```python
from build123d import *

# Parameters (mm, degrees)
HEAD_DEPTH     = 10
SHANK_SKETCH_R = 6
SHANK_DEPTH    = 45
SKETCH6_R      = 7.875
HEAD_CUT_DEPTH = 1.5
FILLET1_R      = 2
FILLET2_R      = 0.5
THREAD_END_W   = 30
THREAD_END_H   = 0.05


with BuildPart() as part:
    # Head Sketch → Head (new body)
    with BuildSketch(Plane.XY):
        Polygon((0, 10.392304845), (9, 5.196152423), (9, -5.196152423), (0, -10.392304845), (-9, -5.196152423), (-9, 5.196152423), align=None)
    extrude(amount=HEAD_DEPTH)

    # Shank Sketch → Shank (add)
    with BuildSketch(Plane.XY):
        Circle(SHANK_SKETCH_R)
    extrude(amount=-SHANK_DEPTH)

    # Sketch3 → Flange (revolve)
    with BuildSketch(Plane(origin=(0, 0, 0), x_dir=(-1, 0, 0), z_dir=(0, 1, 0)), mode=Mode.PRIVATE) as flange_sk:
        with BuildLine():
            Line((-13, 0), (0, 0))
            Line((0, 0), (0, 5))
            ThreePointArc((0, 5), (-6.947778179, 3.955279081), (-13.281081081, 0.913513514))
            ThreePointArc((-13.281081081, 0.913513514), (-13.477889504, 0.352957076), (-13, 0))
        make_face()
    revolve(flange_sk.sketch.rotate(Axis((0, 0, 0), (0, 0, 1)), 30), axis=Axis((0, 0, 0), (0, 0, 1)))

    # Sketch5 → Head Trim (revolve, cut)
    with BuildSketch(Plane(origin=(0, 0, 0), x_dir=(0, 0, -1), z_dir=(1, 0, 0)), mode=Mode.PRIVATE) as head_trim_sk:
        with BuildLine():
            Line((-10, -8.392304845), (-10, -10.392304845))
            Line((-10, -10.392304845), (-8, -10.392304845))
            ThreePointArc((-8, -10.392304845), (-9.414213562, -9.806518408), (-10, -8.392304845))
        make_face()
    revolve(head_trim_sk.sketch.rotate(Axis((0, 0, 15.085599173), (0, 0, -1)), 90), axis=Axis((0, 0, 15.085599173), (0, 0, -1)), mode=Mode.SUBTRACT)

    # Sketch6 → Head Cut (cut)
    with BuildSketch(Plane.XY.offset(10)):
        Circle(SKETCH6_R)
    extrude(amount=-HEAD_CUT_DEPTH, mode=Mode.SUBTRACT)

    # Fillet1
    # the kernel refuses this fillet: 2 mm, written as the material it adds along each edge
    with BuildSketch(Plane(origin=(0, 0, 8.5), x_dir=(1, 0, 0), z_dir=(0, -1, 0))) as fillet1_piece_1:
        with BuildLine():
            CenterArc((5.938508327, 2), FILLET1_R, 270, 75.522487814)
            Line((5.938508327, 0), (5.938508327, -0.04))
            Line((5.938508327, -0.04), (7.875, -0.04))
            Line((7.875, -0.04), (7.915, 0))
            ThreePointArc((7.915, 0), (7.915, 0.75), (7.913729833, 1.49))
            Line((7.913729833, 1.49), (7.875, 1.5))
        make_face()
    revolve(axis=Axis((0, 0, 8.5), (0, 0, 1)))

    # Fillet2
    fillet2_edges = [part.edges().sort_by_distance(p)[0] for p in [
        (-6, 0, 0),
    ]]
    fillet(fillet2_edges, radius=FILLET2_R)

    # Thread End → Thread Cut (revolve, cut)
    with BuildSketch(Plane(origin=(0, 0, 0), x_dir=(0, 0, -1), z_dir=(1, 0, 0)), mode=Mode.PRIVATE) as thread_cut_sk:
        with Locations((30, 5.975)):
            Rectangle(THREAD_END_W, THREAD_END_H)
    revolve(thread_cut_sk.sketch.rotate(Axis((0, 0, -21.551935625), (0, 0, -1)), 90), axis=Axis((0, 0, -21.551935625), (0, 0, -1)), mode=Mode.SUBTRACT)


solid = part.part
```
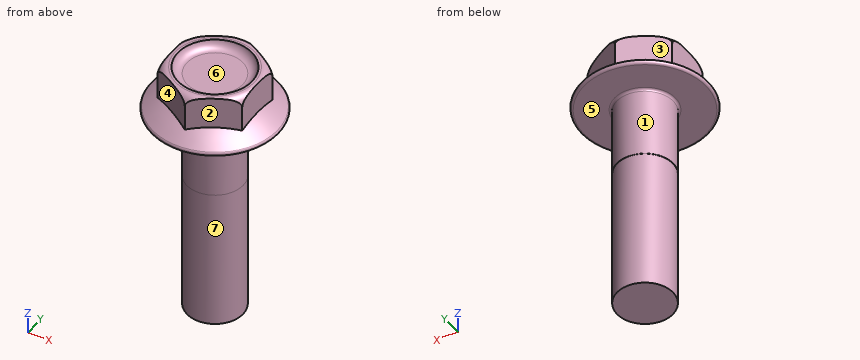
Source: CAD feature listing. Evaluate the final solid. Frame: model axes, mm. Face numbers are marked on the shaded views. A direction names the side the tool comes from. Give positions to 0.01 mm unless a question says otherwise; leave off trailing zeros. Order: outer loops, then holes, each group sorted by start corner. A loop starts at its lowest first (then second) coordinate and runs counter-clockwise, first axis right, second up.
(1) Section query B-B (z = -4). Return the cut outline in (x, y), plus the area to 3 significant figures.
(2) Access query for the marked faces 1, 2, 3 and 4. Directions: +Z, -Z, +X, -X, +Y, -Y. A direction counts if a zero-diameter tool reaches every point of the face in a straight line with its end or side. Return the directions, or none.
(3) Contact query for flat-ended pins moving along their axis: P1, Ø8, axis at x = 3.5, y = -5.5, coming from the -Z side; P2, Ø8, axis at y = -2.5, z = 6.5, coming from the -X side; P3, Ø12, axis at y = 2.5, z = -32, coming from the +X side; P4, Ø2, axis at x = 8.5, z = -15, coming from the +Y side. Output: stop coordinate, or through.
(4) Section query C-C (z = -25.5). Return the cut outline in (x, y), plus the area to 3 significant figures.
(5) Pull-direction query (Y, two-part tool) for the marked faces 5, 6 and 7; classes: +Y half, -Y half, draft (parallel to the pull), parting line (faces both ways), or undercut.
(6) Material intervals for line 1 along X through (y, z) = (0.75, -6.5); line 2 along Z through (x, y) = (0.75, -5.5); line 3 along X through (y, z) = (2, 4.5), sorted ascending.
Outcome:
1. outline: circle Ø12 at (0, 0)
1. area: 113 mm2
2. face 1: -Z
2. face 2: +Z, +X, -Y
2. face 3: +Z, -X, +Y
2. face 4: +Z, -X, -Y
3. P1: stops at z = -45
3. P2: stops at x = -10.33
3. P3: stops at x = 5.95
3. P4: passes through
4. outline: circle Ø11.9 at (0, 0)
4. area: 111 mm2
5. face 5: draft
5. face 6: undercut
5. face 7: parting line
6. line 1: x = -5.95 to 5.95
6. line 2: z = -45 to 8.5
6. line 3: x = -9 to 9
